from build123d import *

# Parameters (mm, degrees)
EXTRUDE_1_DEPTH = 5
EXTRUDE_2_DEPTH = 1


with BuildPart() as part:
    # 草图1 → 凸台-拉伸1 (new, symmetric)
    with BuildSketch(Plane(origin=(0, 0, 0), x_dir=(1, 0, 0), z_dir=(0, 1, 0))):
        with BuildLine():
            Line((0, 0), (4, 0))
            ThreePointArc((4, 0), (2, -2), (0, 0))
        make_face()
    extrude(amount=EXTRUDE_1_DEPTH, both=True)

    # 草图2 → 凸台-拉伸2 (add)
    with BuildSketch(Plane(origin=(0, 5, 0), x_dir=(1, 0, 0), z_dir=(0, 1, 0))):
        with BuildLine():
            Line((-0.5, 0.25), (4.5, 0.25))
            ThreePointArc((4.5, 0.25), (2, -2.25), (-0.5, 0.25))
        make_face()
    extrude(amount=EXTRUDE_2_DEPTH)


solid = part.part
Work out the finished part from the listing and answer in its coordinate system (mm). A direction names the side the tool comes from. Round coordinates to 2 decimals unless told otherwise and drop trailing zeros. Write each loop counter-clockwise with the first axis right and the second up, starting at its lowest first coordinate (ties: lowest second). Pieces come first, ordered by that corner, then holes. Notation, with made-up numbers: (-31.75, -16.5) -> (-21.75, -16.5) arc R14 cw to (-21.75, 7.5) -> close; hole circle Ø7 at (-38, -2). An arc over 180 degrees is marked (long way). Answer as CSV lines item,"result". Start each with the question number.
(1) This flat-tipped pin is pushed along its axis until it touches: pin 1 (3 mm diameter, centred on x = 2, y = 1.5, fed in from -Z). Where does it stop, or does it pass through?
(2) The part is cut by section C-C, the plane y = 1.75. Give the vertices of the cut face in (x, z).
(3) A tool of negligible diameter and unlimited length cuts with its end or side. For faces 1 (the cylindrical face through (2, 0, 2)), 2 (the cylindrical face through (2.05, 5.49, 2.25)), 3 (the flat face through (2, 0, 0)), from which of +Z, -Z, +X, -X, +Y, -Y can it reach the whole face along a straight path? Write none if from no direction.
(4) The part is cut by section A-A, the plane x = 2. Give the vertices of the cut face in (y, z).
(5) The part is cut by section B-B, the plane z = 1.2. Give the vertices of the cut face in (x, y), then the cut area to 3 significant figures.
(6) Find the intervals of material crossed by probe 1 along Y at (x, z) = (-0.1, 0.55); probe 2 along Z at (x, y) = (2, 2.75); probe 3 along X at (y, z) = (3.5, 1.25), in increasing order.
Output values:
1,pin 1,"stops at z = 0"
2,outline,"(0, 0) -> (4, 0) arc R2 ccw to start"
3,face 1,"+Z, -Y"
3,face 2,"+Z, +Y, -Y"
3,face 3,"-Z, +X, -X, -Y"
4,outline,"(-5, 0) -> (5, 0) -> (5, -0.25) -> (6, -0.25) -> (6, 2.25) -> (5, 2.25) -> (5, 2) -> (-5, 2) -> close"
5,outline,"(-0.04, 5) -> (0.4, 5) -> (0.4, -5) -> (3.6, -5) -> (3.6, 5) -> (4.04, 5) -> (4.04, 6) -> (-0.04, 6) -> close"
5,area,"36.1 mm²"
6,probe 1,"y = 5 to 6"
6,probe 2,"z = 0 to 2"
6,probe 3,"x = 0.44 to 3.56"
